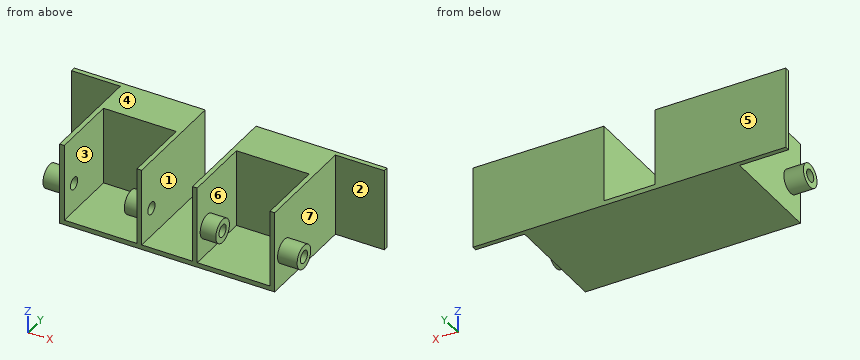
Autodesk Inventor part; units mm, degrees
ref_plane "YZ Plane" through (0, 0, 0) normal (1, 0, 0) x (0, 1, 0)
ref_plane "XZ Plane" through (0, 0, 0) normal (0, 1, 0) x (-1, 0, 0)
ref_plane "XY Plane" through (0, 0, 0) normal (0, 0, 1) x (1, 0, 0)
sketch "Sketch1" plane through (0, 0, 0) normal (0, 0, 1) x (1, 0, 0)
  line L0 (0, 0) -> (110, 0)
  line L1 (110, 0) -> (110, -56)
  line L2 (110, -56) -> (0, -56)
  line L3 (0, -56) -> (0, 0)
  line L4 (0, 0) -> (-25, 0)
  line L5 (-25, 0) -> (-25, -2.4)
  line L6 (-25, -2.4) -> (0, -2.4)
  line L7 (0, -2.4) -> (0, 0)
  line L8 (110, 0) -> (135, 0)
  line L9 (135, 0) -> (135, -2.4)
  line L10 (135, -2.4) -> (110, -2.4)
  line L11 (110, -2.4) -> (110, 0)
  dimension "d0" = 110
  dimension "d1" = 56
  dimension "d2" = 25
  dimension "d3" = 2.4
  dimension "d4" = 25
  dimension "d5" = 2.4
extrude "Extrusion1" add sketch "Sketch1" along normal blind 42
sketch "Sketch2" plane through (0, 0, 42) normal (0, 0, 1) x (1, 0, 0)
  line L0 (2.4, -2.4) -> (107.6, -2.4)
  line L1 (107.6, -2.4) -> (107.6, -54.7735)
  line L2 (2.4, -54.7735) -> (2.4, -2.4)
  line L3 (110, -56) -> (110, -2.4)
  line L4 (0, -2.4) -> (0, -56)
  line L5 (107.6, -54.7735) -> (107.6, -56)
  line L6 (2.4, -54.7735) -> (2.4, -56)
  line L7 (0, -56) -> (110, -56)
  point P0 (0, 0)
  dimension "d8" = 2.4
  dimension "d9" = 2.4
extrude "Extrusion2" cut sketch "Sketch2" against normal blind 39.6
sketch "Sketch3" plane through (0, 0, 42) normal (0, 0, 1) x (1, 0, 0)
  line L0 (135, 0) -> (-25, 0)
  line L1 (55, 0) -> (68, 0)
  line L2 (55, 0) -> (42, 0)
  line L3 (42, 0) -> (42, -2.4)
  line L4 (2.4, -2.4) -> (107.6, -2.4)
  line L5 (68, -2.4) -> (42, -2.4)
  line L6 (68, -2.4) -> (68, 0)
  point P0 (0, 0)
  dimension "d12" = 13
  dimension "d13" = 13
extrude "Extrusion3" cut sketch "Sketch3" against normal blind 39.6
sketch "Sketch4" plane through (0, 0, 2.4) normal (0, 0, 1) x (1, 0, 0)
  line L0 (2.4, -2.4) -> (42, -2.4)
  line L1 (107.6, -56) -> (2.4, -56)
  line L2 (42, -2.4) -> (39.6, -2.4)
  line L3 (39.6, -2.4) -> (39.6, -56)
  line L4 (39.6, -56) -> (42, -56)
  line L5 (42, -56) -> (42, -2.4)
  line L6 (68, -2.4) -> (107.6, -2.4)
  line L7 (68, -2.4) -> (70.4, -2.4)
  line L8 (70.4, -2.4) -> (70.4, -56)
  line L9 (70.4, -56) -> (68, -56)
  line L10 (68, -56) -> (68, -2.4)
  point P0 (0, 0)
  dimension "d16" = 2.4
  dimension "d17" = 2.4
extrude "Extrusion4" add sketch "Sketch4" along normal blind 39.6
sketch "Sketch5" plane through (-25, -2.4, 0) normal (0, -1, 0) x (1, 0, 0)
  circle A0 centre (12.5, 30) radius 1.5
  circle A1 centre (12.5, 12) radius 1.5
  line L0 (0, 42) -> (25, 42)
  line L1 (0, 0) -> (25, 0)
  dimension "d20" = 3
  dimension "d21" = 3
  dimension "d22" = 12
  dimension "d23" = 12
sketch "Sketch6" plane through (2.4, -2.4, 2.4) normal (0, -1, 0) x (1, 0, 0)
  line L0 (37.2, 0) -> (37.2, 39.6)
  line L1 (0, 39.6) -> (37.2, 39.6)
  line L2 (37.2, 39.6) -> (37.2, 0)
  line L3 (37.2, 0) -> (0, 0)
  line L4 (0, 0) -> (0, 39.6)
  line L5 (68, 39.6) -> (68, 0)
  line L6 (105.2, 39.6) -> (105.2, 0)
  line L7 (68, 39.6) -> (105.2, 39.6)
  line L8 (105.2, 39.6) -> (105.2, 0)
  line L9 (105.2, 0) -> (68, 0)
  line L10 (68, 0) -> (68, 39.6)
  point P0 (-2.4, -2.4)
extrude "Extrusion5" add sketch "Sketch6" along normal blind 19
sketch "Sketch7" plane through (0, -56, 0) normal (-1, 0, 0) x (0, 0, 1)
  circle A0 centre (17, 8.6) radius 3.15
  line L0 (0, 53.6) -> (0, 0)
  line L1 (0, 53.6) -> (42, 53.6)
  point P0 (0, 56)
  dimension "d26" = 6.3
  dimension "d27" = 17
  dimension "d28" = 45
extrude "Extrusion6" cut sketch "Sketch7" against normal blind 110
sketch "Sketch8" plane through (0, -56, 0) normal (-1, 0, 0) x (0, 0, 1)
  circle A0 centre (17, 8.6) radius 3.15
  circle A1 centre (17, 8.6) radius 6
  point P0 (0, 56)
  dimension "d31" = 12
extrude "Extrusion7" add sketch "Sketch8" along normal blind 10
sketch "Sketch9" plane through (39.6, -56, 2.4) normal (-1, 0, 0) x (0, 0, 1)
  circle A0 centre (14.6, 8.6) radius 3.15
  circle A1 centre (14.6, 8.6) radius 6
  point P0 (-2.4, 56)
  dimension "d34" = 12
extrude "Extrusion8" add sketch "Sketch9" along normal blind 8
sketch "Sketch10" plane through (110, -56, 0) normal (1, 0, 0) x (0, 0, -1)
  circle A0 centre (-17, 8.6) radius 3.15
  circle A1 centre (-17, 8.6) radius 6
  point P0 (0, 56)
  dimension "d37" = 12
extrude "Extrusion9" add sketch "Sketch10" along normal blind 10
sketch "Sketch11" plane through (70.4, -56, 42) normal (1, 0, 0) x (0, 0, -1)
  circle A0 centre (25, 8.6) radius 3.15
  circle A1 centre (25, 8.6) radius 6
  point P0 (42, 56)
  dimension "d40" = 12
extrude "Extrusion10" add sketch "Sketch11" along normal blind 8
sketch "Sketch12" plane through (2.4, -21.4, 2.4) normal (0, -1, 0) x (1, 0, 0)
  circle A0 centre (22.2, 14.6) radius 13.25
  circle A1 centre (83, 14.6) radius 13.25
  line L0 (68, 0) -> (68, 39.6)
  line L1 (37.2, 0) -> (37.2, 39.6)
  line L2 (37.2, 39.6) -> (0, 39.6)
  line L3 (105.2, 39.6) -> (68, 39.6)
  point P0 (-2.4, -2.4)
  dimension "d43" = 26.5
  dimension "d44" = 26.5
  dimension "d45" = 15
  dimension "d46" = 15
  dimension "d47" = 25
  dimension "d48" = 25
properties part number "Chassi_Rear"
Can you work these out from the model? Positions are in its coordinate system, mm. Face numbers are marked on the shaded views. A direction names the side the tool comes from. Give positions to 0.01 mm unless a question says otherwise; leave off trailing zeros. Order: outer loops, then holes, each group sorted by start corner. A loop starts at its lowest first (then second) coordinate and runs counter-clockwise, first axis right, second up. Notation, with made-up numbers: M 69.25,-1 L 85.25,-1 A28 ccw 85.25,31 Z; hole C 53,-13 d10. An arc over 180 degrees is marked long. One line per item, written item: value.
Item 1: Please list where these lines run through material, in increasing order: line 1 (X direction, y = -47, z = 26); line 2 (Y direction, x = 72, z = 17); line 3 (X direction, y = -5, z = 34).
Verdict:
line 1: 0 to 2.4, 39.6 to 42, 68 to 70.4, 107.6 to 110
line 2: -53.4 to -50.55, -44.25 to -41.4, -21.4 to 0
line 3: 0 to 42, 68 to 110
Item 2: If we section it at B-B on y = -47.4: State how many separate pieces and enclosed holes the cut face has, and give its area (3 significant figures).
Verdict:
separate pieces: 5
enclosed holes: 0
area: 789 mm2
Item 3: If we section it at A-A on z = 28: Write out the boundary of the cut face in (x, y), and give its area (3 significant figures).
Verdict:
outline: M -25,-2.4 L 0,-2.4 L 0,-56 L 2.4,-56 L 2.4,-21.4 L 39.6,-21.4 L 39.6,-56 L 42,-56 L 42,0 L -25,0 Z; M 68,-56 L 70.4,-56 L 70.4,-21.4 L 107.6,-21.4 L 107.6,-56 L 110,-56 L 110,-2.4 L 135,-2.4 L 135,0 L 68,0 Z
area: 2,250 mm2
Item 4: For pin 1 (20 mm diameter, centred on y = -39.5, z = 25.5, fed in from +X); pin 2 (10.5 mm diameter, centred on y = -34.5, z = 26, fed in from +X); pin 3 (6 mm diameter, centred on y = -49, z = 20, fed in from -X), each with a flat end and sliding along its axis, tell me the tip position at first contact or that it passes through.
Verdict:
pin 1: x = 120
pin 2: x = 110
pin 3: x = -10
Item 5: If we mould it in two halves opening along Y, with no side actions, what happens to the marked faces 4, 5, 6 and 7? For each: pulls with the +Y half, pulls with the -Y half, needs draft (parallel to the pull), parting line crosses it, or undercut.
Verdict:
face 4: needs draft
face 5: pulls with the +Y half
face 6: undercut
face 7: undercut
Item 6: If we section it at C-C on x = 23: Write out the boundary of the cut face in (y, z), and give its area (3 significant figures).
Verdict:
outline: M -56,0 L 0,0 L 0,42 L -21.4,42 L -21.4,2.4 L -56,2.4 Z
area: 982 mm2
Item 7: For the marked faces 1, 2 and 3, which set-ups out of +Z, -Z, +X, -X, +Y, -Y let a thin tool reach every point of the face, with its end or its side?
Verdict:
face 1: +Z, +Y, -Y
face 2: +Z, -Z, +X
face 3: +Z, -Y
Item 8: If we section it at D-D on y = -14: Write out the boundary of the cut face in (x, z), and give its area (3 significant figures).
Verdict:
outline: M 0,0 L 110,0 L 110,42 L 68,42 L 68,2.4 L 42,2.4 L 42,42 L 0,42 Z
area: 3,590 mm2
